Check sheet for the modelled part. Datum: model origin and axes. Units: mm. Face numbers are marked on the shaded views. Give positions to 0.01 mm unless a question says otherwise; leave off trailing zeros. Write each loop counter-clockwise with the first axis right and the second up, starting at its lowest first coordinate (ties: lowest second). Pieces come first, ordered by that corner, then holes. Notation, with made-up numbers: (87.25, 82) -> (136.25, 82) arc R19 ccw to (136.25, 99) -> close; hole circle Ø7 at (29.5, 87.25). An arc over 180 degrees is marked (long way). Return JSON: item names as keys, results as strings.
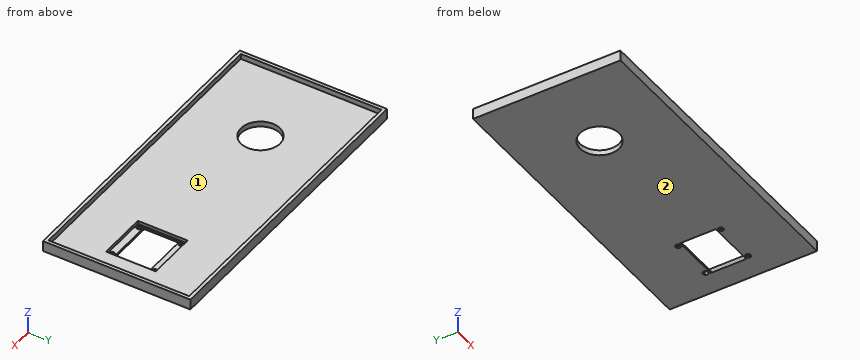
Autodesk Fusion 360 part; units mm, degrees
sketch "Sketch1" plane through (0, 0, 0) normal (0, 0, 1) x (1, 0, 0)
  line L0 (76.5, 41.5) -> (-76.5, 41.5)
  line L1 (-76.5, 41.5) -> (-76.5, -41.5)
  line L2 (-76.5, -41.5) -> (76.5, -41.5)
  line L3 (76.5, -41.5) -> (76.5, 41.5)
  line L4 (76.5, 41.5) -> (-76.5, -41.5) construction
  line L5 (-76.5, 41.5) -> (76.5, -41.5) construction
  dimension "d1" = 153
  dimension "d2" = 83
extrude "Extrude1" add sketch "Sketch1" along normal blind 3
sketch "Sketch2" plane through (0, 0, 3) normal (0, 0, 1) x (-1, 0, 0)
  line L0 (-76.5, 41.5) -> (-76.5, -41.5)
  line L1 (-76.5, -41.5) -> (76.5, -41.5)
  line L2 (76.5, -41.5) -> (76.5, 41.5)
  line L3 (76.5, 41.5) -> (-76.5, 41.5)
  line L4 (-74.6, -39.6) -> (74.6, -39.6)
  line L5 (74.6, -39.6) -> (74.6, 39.6)
  line L6 (74.6, 39.6) -> (-74.6, 39.6)
  line L7 (-74.6, 39.6) -> (-74.6, -39.6)
  dimension "d5" = -1.9
extrude "Extrude2" add sketch "Sketch2" along normal blind 3
sketch "Sketch3" plane through (-76.5, 0, 0) normal (-1, 0, 0) x (0, -1, 0)
  line L0 (-41.5, 0) -> (41.5, 0)
  line L1 (41.5, 0) -> (41.5, 6)
  line L2 (41.5, 6) -> (-41.5, 6)
  line L3 (-41.5, 6) -> (-41.5, 0)
sketch "Sketch4" plane through (0, 0, 0) normal (0, 1, 0) x (1, 0, 0)
sketch "Sketch5" plane through (0, 0, 3) normal (0, 0, 1) x (-1, 0, 0)
  line L0 (-74.6, -39.6) -> (74.6, -39.6)
  line L1 (74.6, -39.6) -> (74.6, 39.6)
  line L2 (74.6, 39.6) -> (-74.6, 39.6)
  line L3 (-74.6, 39.6) -> (-74.6, -39.6)
  line L4 (-36.5, 10) -> (-63.5, 10)
  line L5 (-63.5, 10) -> (-63.5, -10)
  line L6 (-63.5, -10) -> (-36.5, -10)
  line L7 (-36.5, -10) -> (-36.5, 10)
  line L8 (-36.5, 10) -> (-63.5, -10) construction
  line L9 (-63.5, 10) -> (-36.5, -10) construction
  line L10 (-36, -14) -> (-64, -14)
  line L11 (-64, -14) -> (-64, 14)
  line L12 (-64, 14) -> (-36, 14)
  line L13 (-36, 14) -> (-36, -14)
  line L14 (-36, -14) -> (-64, 14) construction
  line L15 (-64, -14) -> (-36, 14) construction
  circle A0 centre (-37.9567, 12.0433) radius 1.5
  circle A1 centre (-61.9549, 11.9549) radius 1.5
  circle A2 centre (-62.1598, -12.1598) radius 1.5
  circle A3 centre (-37.9351, -12.0649) radius 1.5
  point P0 (-50, 0)
  point P1 (-50, 0)
  dimension "d8" = 27
  dimension "d9" = 20
  dimension "d12" = 28
  dimension "d13" = 28
  dimension "d14" = 3
  dimension "d15" = 3
  dimension "d16" = 3
  dimension "d17" = 3
extrude "Extrude3" cut sketch "Sketch5" against normal blind 3 contours L4 L5 L6 L7
extrude "Extrude4" cut sketch "Sketch5" against normal blind 4 contours A0
extrude "Extrude5" cut sketch "Sketch5" against normal blind 4 contours A1
extrude "Extrude6" cut sketch "Sketch5" against normal blind 4 contours A2
extrude "Extrude7" cut sketch "Sketch5" against normal blind 5 contours A3
extrude "Extrude8" cut sketch "Sketch5" against normal blind 1.8 contours L10 L11 L12 L13
extrude "Extrude9" add sketch "Sketch3" along normal blind 20
move_face "OffsetFaces1" offset -20 1 faces at (-74.6, 13.2, 5)
sketch "Sketch6" plane through (0, 0, 3) normal (0, 0, 1) x (-1, 0, 0)
  circle A0 centre (50, 0) radius 11
  dimension "d31" = 22
extrude "Extrude10" cut sketch "Sketch6" against normal blind 5
(1) Cross-section at A-A on z = 4.1. Enter the section's corners in (x, y), then the cut area to 3 significant figures.
Reply:
{"outline": "(-96.5, -41.5) -> (76.5, -41.5) -> (76.5, 41.5) -> (-96.5, 41.5) -> close; hole (-94.6, -39.6) -> (74.6, -39.6) -> (74.6, 39.6) -> (-94.6, 39.6) -> close", "area": "958 mm^2"}
(2) Cross-section at C-C on x = -50. Enter the section's corners in (y, z).
Reply:
{"outline": "(-41.5, 0) -> (-11, 0) -> (-11, 3) -> (-39.6, 3) -> (-39.6, 6) -> (-41.5, 6) -> close; (11, 0) -> (41.5, 0) -> (41.5, 6) -> (39.6, 6) -> (39.6, 3) -> (11, 3) -> close"}
(3) Cross-section at B-B on y = 26.5. Enter the section's corners in (x, z).
Reply:
{"outline": "(-96.5, 0) -> (76.5, 0) -> (76.5, 6) -> (74.6, 6) -> (74.6, 3) -> (-94.6, 3) -> (-94.6, 6) -> (-96.5, 6) -> close"}
(4) Depth check by flat-ended pin: pin 1 Ø24 at (x, y) = (-45, 8) entering from +Z. Enter the tip coordinate at first touch or a pass-through.
Reply:
{"pin 1": "z = 3"}
(5) Cross-section at D-D on y = 7. Enter the section's corners in (x, z), then the cut area to 3 significant figures.
Reply:
{"outline": "(-96.5, 0) -> (-58.49, 0) -> (-58.49, 3) -> (-94.6, 3) -> (-94.6, 6) -> (-96.5, 6) -> close; (-41.51, 0) -> (36.5, 0) -> (36.5, 1.2) -> (36, 1.2) -> (36, 3) -> (-41.51, 3) -> close; (63.5, 0) -> (76.5, 0) -> (76.5, 6) -> (74.6, 6) -> (74.6, 3) -> (64, 3) -> (64, 1.2) -> (63.5, 1.2) -> close", "area": "397 mm^2"}
(6) Thickness scan on L1, parallel to Y at x = -72, z = 3.4; L2, parallel to X at y = 25.5, z = 3.5; L3, parallel to X at y = -9.5, z = 1.8. Record the ranges inside material, lowest first.
Reply:
{"L1": "-41.5 to -39.6, 39.6 to 41.5", "L2": "-96.5 to -94.6, 74.6 to 76.5", "L3": "-96.5 to -55.55, -44.45 to 36, 64 to 76.5"}
(7) Release check for a two-part mould opening along Y. For the marked faces 1 and 2 record: pulls with the +Y half, pulls with the -Y half, needs draft (parallel to the pull), parting line crosses it, or undercut.
Reply:
{"face 1": "undercut", "face 2": "needs draft"}
